Can you work these out from the model? Positions are in its coordinate system, mm. Face numbers are marked on the shaded views. Round coordinates to 2 decimals unless told otherwise and drop trailing zeros. Loops run counter-clockwise (first coordinate to the right, second up) from the corner with the lowest first, then second, coordinate; pieces in that order, holes last.
(1) I want a section at B-B on x = 38. Write out the boundary of the cut face in (y, z) (3 decimals).
(2) I want a section at A-A on z = 2.5. Write out the boundary of the cut face in (x, y) (3 decimals).
(3) If I drill on line 1 along X through (y, z) = (5, -18); line 2 along Y through (x, z) = (29, 9); line 3 along Z through (x, y) = (-18.5, 9), over which ranges is the centre line in solid material (lowest first)?
(4) I want a section at C-C on z = -20.5. Write out the boundary of the cut face in (x, y) (3 decimals).
(5) Thinking about a two-plate mould opening in Z: for the marked faces 1, 2 and 3, which applies, released by +Z, released by -Z, zero draft, split by the parting line, or undercut?
(6) Will this pin go through, and if not, where does the flat tip stop? pin 1 Ø2 at (y, z) = (3.5, 2.5) entering from -X.
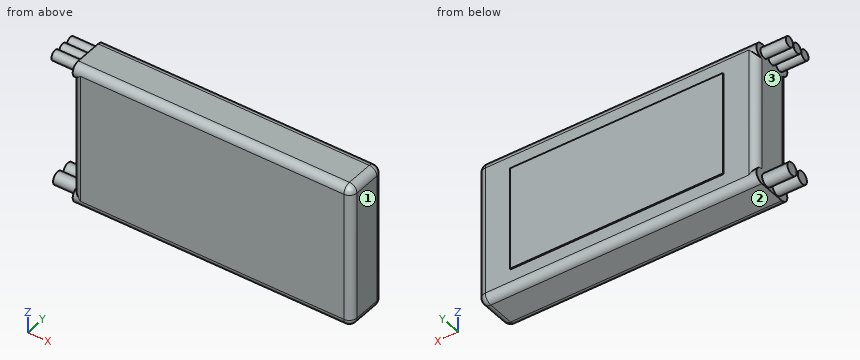
from build123d import *

# Parameters (mm, degrees)
SKETCH1_W       = 69.85
SKETCH1_H       = 36.068
BATTERY_DEPTH   = 10.668
FILLET_2_R      = 1.905
WIRE_BOSS_DEPTH = 5.08
SKETCH3_R       = 1.27
SKETCH3_R_2     = 1.5875
WIRES_2_DEPTH   = 6.35
SKETCH4_W       = 53.34
SKETCH4_H       = 25.908
LABEL_DEPTH     = 0.254


with BuildPart() as part:
    # Sketch1 → Battery (new body)
    with BuildSketch(Plane(origin=(0, 0, 0), x_dir=(1, 0, 0), z_dir=(0, 1, 0))):
        with Locations((8.399917755, 5.125761329)):
            Rectangle(SKETCH1_W, SKETCH1_H)
    extrude(amount=BATTERY_DEPTH)

    # Fillet 2
    fillet_2_edges = [part.edges().sort_by_distance(p)[0] for p in [
        (43.324917755, 10.668, -5.125761329),
        (8.399917755, 10.668, -23.159761329),
        (-26.525082245, 10.668, -5.125761329),
        (8.399917755, 0, -23.159761329),
        (43.324917755, 0, -5.125761329),
        (8.399917755, 0, 12.908238671),
        (-26.525082245, 0, -5.125761329),
        (8.399917755, 10.668, 12.908238671),
        (-26.525082245, 5.334, -23.159761329),
        (43.324917755, 5.334, -23.159761329),
        (43.324917755, 5.334, 12.908238671),
        (-26.525082245, 5.334, 12.908238671),
    ]]
    fillet(fillet_2_edges, radius=FILLET_2_R)

    # Sketch2 → Wire Boss (add)
    with BuildSketch(Plane.ZY.offset(26.525082245)):
        with BuildLine():
            Line((12.908238671, 8.763), (12.908238671, 1.905))
            ThreePointArc((12.908238671, 1.905), (11.003238671, 0), (9.098238671, 1.905))
            Line((9.098238671, 1.905), (9.098238671, 8.763))
            ThreePointArc((9.098238671, 8.763), (11.003238671, 10.668), (12.908238671, 8.763))
        make_face()
        with BuildLine():
            Line((-19.349761329, 8.763), (-19.349761329, 1.905))
            ThreePointArc((-19.349761329, 1.905), (-21.254761329, 0), (-23.159761329, 1.905))
            Line((-23.159761329, 1.905), (-23.159761329, 8.763))
            ThreePointArc((-23.159761329, 8.763), (-21.254761329, 10.668), (-19.349761329, 8.763))
        make_face()
    extrude(amount=-WIRE_BOSS_DEPTH)

    # Sketch3 → Wires 2 (add)
    with BuildSketch(Plane.ZY.offset(26.525082245)):
        with Locations((11.003238671, 8.001)):
            Circle(SKETCH3_R)
        with Locations((11.003238671, 5.334)):
            Circle(SKETCH3_R)
        with Locations((11.003238671, 2.667)):
            Circle(SKETCH3_R)
        with Locations((-21.254761329, 7.112)):
            Circle(SKETCH3_R_2)
        with Locations((-21.254761329, 3.556)):
            Circle(SKETCH3_R_2)
    extrude(amount=WIRES_2_DEPTH)

    # Sketch4 → Label (add)
    with BuildSketch(Plane(origin=(0, 10.668, 0), x_dir=(1, 0, 0), z_dir=(0, 1, 0))):
        with Locations((8.399917755, 5.125761329)):
            Rectangle(SKETCH4_W, SKETCH4_H)
    extrude(amount=LABEL_DEPTH)


solid = part.part
Filled sheet:
1. outline: (0, -21.255) arc R1.905 ccw to (1.905, -23.16) - (8.763, -23.16) arc R1.905 ccw to (10.668, -21.255) - (10.668, 11.003) arc R1.905 ccw to (8.763, 12.908) - (1.905, 12.908) arc R1.905 ccw to (0, 11.003) - close
2. outline: (-26.525, 1.905) arc R1.905 ccw to (-24.62, 0) - (41.42, 0) arc R1.905 ccw to (43.325, 1.905) - (43.325, 8.763) arc R1.905 ccw to (41.42, 10.668) - (35.07, 10.668) - (35.07, 10.922) - (-18.27, 10.922) - (-18.27, 10.668) - (-24.62, 10.668) arc R1.905 ccw to (-26.525, 8.763) - close
3. line 1: x = -26.53 to 43.32
3. line 2: y = 0 to 10.67
3. line 3: z = -23.14 to 12.89
4. outline: (-32.875, 2.159) - (-26.525, 2.159) - (-26.525, 0.156) - (-25.375, 0.156) arc R1.905 ccw to (-24.62, 0) - (41.42, 0) arc R1.905 ccw to (43.325, 1.905) - (43.325, 8.763) arc R1.905 ccw to (41.42, 10.668) - (-24.62, 10.668) arc R1.905 ccw to (-25.375, 10.512) - (-26.525, 10.512) - (-26.525, 8.509) - (-32.875, 8.509) - (-32.875, 5.715) - (-26.525, 5.715) - (-26.525, 4.953) - (-32.875, 4.953) - close
5. face 1: zero draft
5. face 2: released by -Z
5. face 3: undercut
6. pin 1: stops at x = -26.53
